from build123d import *

# Parameters (mm, degrees)
F0_W      = 50
F0_H      = 16
F1_DEPTH  = 4
F2_W      = 95
F2_H      = 23
F3_DEPTH  = 33
F4_W      = 13
F4_H      = 23
F5_DEPTH  = 17
F6_DEPTH  = 14
F7_DEPTH  = 14
F8_W      = 13
F8_H      = 5
F8_W_2    = 12.8848927021
F9_DEPTH  = 3
F10_W     = 50
F10_H     = 16
F11_DEPTH = 4
F13_DEPTH = 20
F15_DEPTH = 33
F17_DEPTH = 14
F18_DEPTH = 17
F19_W     = 13
F19_H     = 5
F20_DEPTH = 3
F21_R     = 1.5
F22_DEPTH = 23.001
F23_W     = 5
F23_H     = 10
F24_DEPTH = 38
F25_W     = 22
F25_H     = 5
F25_R     = 1
F26_DEPTH = 2


with BuildPart() as f1:
    # F0 (on Front) → F1 (new body)
    with BuildSketch(Plane.XZ):
        Rectangle(F0_W, F0_H)
    extrude(amount=F1_DEPTH)

    # F2 (on face) → F3 (join)
    with BuildSketch(Plane.XZ.offset(4)):
        Rectangle(F2_W, F2_H)
    extrude(amount=F3_DEPTH)

    # F4 (on face) → F5 (cut)
    with BuildSketch(Plane.XY.offset(11.5)):
        with Locations((0, -20.5)):
            Rectangle(F4_W, F4_H)
    extrude(amount=-F5_DEPTH, mode=Mode.SUBTRACT)

    # F4 (on face) → F6 (cut)
    with BuildSketch(Plane.XY.offset(11.5)):
        Polygon((-29.5, -9), (-35.269472748, -9), (-42.5, -9), (-42.5, -21.713828668), (-42.5, -32), (-35.5076789856, -32), (-29.5, -32), (-29.5, -21.9520311803), align=None)
    extrude(amount=-F6_DEPTH, mode=Mode.SUBTRACT)

    # F4 (on face) → F7 (cut)
    with BuildSketch(Plane.XY.offset(11.5)):
        Polygon((42.4793356239, -31.9733636137), (42.3848927021, -9), (29.5, -9), (29.5, -22.5475411862), (29.5, -32.026721337), (36, -32), align=None)
    extrude(amount=-F7_DEPTH, mode=Mode.SUBTRACT)

    # F8 (on face) → F9 (join)
    with BuildSketch(Plane.XY.offset(11.5)):
        with Locations((-36, -6.5)):
            Rectangle(F8_W, F8_H)
        with Locations((-36, -34.5)):
            Rectangle(F8_W, F8_H)
        with Locations((35.9424463511, -6.5)):
            Rectangle(F8_W_2, F8_H)
        Polygon((29.5, -32.026721337), (29.5204450239, -37), (42.5, -37), (42.4793356239, -31.9733636137), align=None)
    extrude(amount=F9_DEPTH)

    # F10 (on face) → F11 (cut, through all)
    with BuildSketch(Plane(origin=(0, 0, 0), x_dir=(-1, 0, 0), z_dir=(0, 1, 0))):
        Rectangle(F10_W, F10_H)
    extrude(amount=-F11_DEPTH, mode=Mode.SUBTRACT)

    # F12 (on face) → F13 (join)
    with BuildSketch(Plane(origin=(0, -4, 0), x_dir=(-1, 0, 0), z_dir=(0, 1, 0))):
        Polygon((22.5, 9.5), (22.5, 11.5), (0, 11.5), (-22.5, 11.5), (-22.5, 9.5), align=None)
    extrude(amount=F13_DEPTH)

    # F14 (on face) → F15 (join)
    with BuildSketch(Plane.XZ.offset(37)):
        Polygon((-29.5, -11.5), (0, -11.5), (29.5, -11.5), (29.5204450239, 11.5), (-29.5, 11.5), align=None)
    extrude(amount=F15_DEPTH)

    # F16 (on face) → F17 (cut)
    with BuildSketch(Plane.XY.offset(11.5)):
        Polygon((-24.5, -65), (-17.6737755537, -65), (-11.5, -65), (-11.5, -54.9432039261), (-11.5, -42), (-18.178511411, -42), (-24.5, -42), (-24.5, -55.7003095746), align=None)
    extrude(amount=-F17_DEPTH, mode=Mode.SUBTRACT)

    # F16 (on face) → F18 (cut)
    with BuildSketch(Plane.XY.offset(11.5)):
        Polygon((24.5204450239, -42), (17.1529948711, -42), (11.5, -42), (11.5, -54.9432039261), (11.5, -65), (19.4243043661, -65), (24.5204450239, -65), (24.5204450239, -53.5), align=None)
    extrude(amount=-F18_DEPTH, mode=Mode.SUBTRACT)

    # F19 (on face) → F20 (join)
    with BuildSketch(Plane.XY.offset(11.5)):
        with Locations((-18, -67.5)):
            Rectangle(F19_W, F19_H)
        with Locations((-18, -39.5)):
            Rectangle(F19_W, F19_H)
    extrude(amount=F20_DEPTH)

    # F21 (on face) → F22 (cut, through all)
    with BuildSketch(Plane.XY.offset(11.5)):
        with Locations((-12, 8)):
            Circle(F21_R)
        with Locations((12, 8)):
            Circle(F21_R)
    extrude(amount=-F22_DEPTH, mode=Mode.SUBTRACT)

    # F23 (on face) → F24 (cut, through all)
    with BuildSketch(Plane.XZ.offset(70)):
        with Locations((-18, -6.3054482453)):
            Rectangle(F23_W, F23_H)
        with Locations((0, -6.3054482453)):
            Rectangle(F23_W, F23_H)
        with Locations((18.0102225119, -6.3054482453)):
            Rectangle(F23_W, F23_H)
        with Locations((-36, -6.3054482453)):
            Rectangle(F23_W, F23_H)
        with Locations((36, -6.3054482453)):
            Rectangle(F23_W, F23_H)
    extrude(amount=-F24_DEPTH, mode=Mode.SUBTRACT)

    # F25 (on face) → F26 (join)
    with BuildSketch(Plane(origin=(0, 16, 0), x_dir=(-1, 0, 0), z_dir=(0, 1, 0))):
        with Locations((0, 14)):
            Rectangle(F25_W, F25_H)
        with Locations((-8, 14)):
            Circle(F25_R, mode=Mode.SUBTRACT)
        with Locations((-4, 14)):
            Circle(F25_R, mode=Mode.SUBTRACT)
        with Locations((0, 14)):
            Circle(F25_R, mode=Mode.SUBTRACT)
        with Locations((4, 14)):
            Circle(F25_R, mode=Mode.SUBTRACT)
        with Locations((8, 14)):
            Circle(F25_R, mode=Mode.SUBTRACT)
    extrude(amount=-F26_DEPTH)


solid = f1.part
Read the model definition and answer for the solid it produces. Units are mm, in the model's axes. A direction names the side the tool comes from. Give positions to 0.01 mm unless a question says otherwise; leave off trailing zeros. Loops run counter-clockwise (first coordinate to the right, second up) from the corner with the lowest first, then second, coordinate; pieces in that order, holes last. Notation, with made-up numbers: (-8.75, -8) -> (43.25, -8) arc R23 ccw to (43.25, 10) -> close; hole circle Ø7 at (56, 12). An arc over 180 degrees is marked (long way). Use a Markdown table: item, result.
Q1. Section A-A, the plane y = 8 is taken. Determine the outline of the cut face in (x, z), then the cut area to 3 significant figures.
Solved:
| item | result |
|---|---|
| outline | (-22.5, 9.5) -> (-13.5, 9.5) -> (-13.5, 11.5) -> (-22.5, 11.5) -> close; (-10.5, 9.5) -> (10.5, 9.5) -> (10.5, 11.5) -> (-10.5, 11.5) -> close; (13.5, 9.5) -> (22.5, 9.5) -> (22.5, 11.5) -> (13.5, 11.5) -> close |
| area | 78.0 mm^2 |
Q2. Section C-C, the plane z = 7.25 is taken. Determine the outline of the cut face in (x, y), then the cut area to 3 significant figures.
Solved:
| item | result |
|---|---|
| outline | (-47.5, -37) -> (-29.5, -37) -> (-29.5, -70) -> (29.52, -70) -> (29.52, -37) -> (47.5, -37) -> (47.5, -4) -> (-47.5, -4) -> close; hole (-42.5, -32) -> (-29.5, -32) -> (-29.5, -9) -> (-42.5, -9) -> close; hole (-24.5, -65) -> (-11.5, -65) -> (-11.5, -42) -> (-24.5, -42) -> close; hole (-6.5, -32) -> (6.5, -32) -> (6.5, -9) -> (-6.5, -9) -> close; hole (11.5, -65) -> (24.52, -65) -> (24.52, -42) -> (11.5, -42) -> close; hole (29.5, -32.03) -> (42.48, -31.97) -> (42.38, -9) -> (29.5, -9) -> close |
| area | 3,590 mm^2 |
Q3. Section D-D, the plane y = -26.5 is taken. Determine the outline of the cut face in (x, z).
Solved:
| item | result |
|---|---|
| outline | (-47.5, -11.5) -> (47.5, -11.5) -> (47.5, 11.5) -> (42.46, 11.5) -> (42.46, -2.5) -> (29.5, -2.5) -> (29.5, 11.5) -> (6.5, 11.5) -> (6.5, -5.5) -> (-6.5, -5.5) -> (-6.5, 11.5) -> (-29.5, 11.5) -> (-29.5, -2.5) -> (-42.5, -2.5) -> (-42.5, 11.5) -> (-47.5, 11.5) -> close |
Q4. A tool of negligible diameter and unlimited length cuts with its end or side. For faces 1 (the face through (-36, -20, -2.5)), 2 (the face through (-29.5, -35, 13)), 3 (the face through (0, -51, -1.305)), from which of +Z, -Z, +X, -X, +Y, -Y can it reach the whole face along a straight path? Write none if from no direction.
Solved:
| item | result |
|---|---|
| face 1 | +Z |
| face 2 | +Z, +Y, -Y |
| face 3 | -Y |
Q5. Each of these flat-tipped pins is pushed along its axis until it touches: pin 1 (1 mm diameter, centred on x = -29.5, z = 6, fed in from +Y); pin 2 (5.5 mm diameter, centred on x = -20, y = -39, fed in from +Z); pin 3 (12 mm diameter, centred on x = 4, y = -53.5, fed in from +Z). Where does it stop, or does it pass through?
Solved:
| item | result |
|---|---|
| pin 1 | stops at y = -4 |
| pin 2 | stops at z = 14.5 |
| pin 3 | stops at z = 11.5 |
Q6. Determine the mould class of faces 4 (the face through (36, -35, -11.305)), 5 (the face through (-29.5, -53, 0)), 6 (the face through (38.5, -35, -6)), 7 (the face through (45, -20, 11.5)) for opening direction Z: pulls with the +Z half, pulls with the -Z half, needs draft (parallel to the pull), parting line crosses it, or undercut.
Solved:
| item | result |
|---|---|
| face 4 | undercut |
| face 5 | needs draft |
| face 6 | undercut |
| face 7 | pulls with the +Z half |
Q7. Section B-B, the plane y = -57 is taken. Determine the outline of the cut face in (x, z), then the cut area to 3 significant figures.
Solved:
| item | result |
|---|---|
| outline | (-29.5, -11.5) -> (29.5, -11.5) -> (29.52, 11.5) -> (24.52, 11.5) -> (24.52, -5.5) -> (20.51, -5.5) -> (20.51, -11.31) -> (15.51, -11.31) -> (15.51, -5.5) -> (11.5, -5.5) -> (11.5, 11.5) -> (-11.5, 11.5) -> (-11.5, -2.5) -> (-15.5, -2.5) -> (-15.5, -11.31) -> (-20.5, -11.31) -> (-20.5, -2.5) -> (-24.5, -2.5) -> (-24.5, 11.5) -> (-29.5, 11.5) -> close; hole (-2.5, -11.31) -> (2.5, -11.31) -> (2.5, -1.31) -> (-2.5, -1.31) -> close |
| area | 831 mm^2 |
Q8. Find the intervals of material crossed by line 1 along Y through (x, z) = (12, 10.6); line 2 along X through (y, z) = (-55, -4.5); line 3 along X through (y, z) = (-44.5, 4.75), in increasing order.
Solved:
| item | result |
|---|---|
| line 1 | y = -70 to -65, -42 to 6.5, 9.5 to 16 |
| line 2 | x = -29.5 to -20.5, -15.5 to -2.5, 2.5 to 11.5, 24.52 to 29.51 |
| line 3 | x = -29.5 to -24.5, -11.5 to 11.5, 24.52 to 29.51 |
